Autodesk Inventor part; units mm, degrees
ref_plane "YZ Plane" through (0, 0, 0) normal (1, 0, 0) x (0, 1, 0)
ref_plane "XZ Plane" through (0, 0, 0) normal (0, 1, 0) x (-1, 0, 0)
ref_plane "XY Plane" through (0, 0, 0) normal (0, 0, 1) x (1, 0, 0)
sketch "스케치1" plane through (0, 0, 0) normal (0, 0, 1) x (1, 0, 0)
  line L0 (27.7299, -18.5773) -> (-27.7299, -18.5773)
  line L1 (-27.7299, -18.5773) -> (-27.7299, 18.5773)
  line L2 (-27.7299, 18.5773) -> (27.7299, 18.5773)
  line L3 (27.7299, 18.5773) -> (27.7299, -18.5773)
  line L4 (27.7299, -18.5773) -> (-27.7299, 18.5773) construction
  line L5 (-27.7299, -18.5773) -> (27.7299, 18.5773) construction
  point P0 (0, 0)
extrude "돌출1" add sketch "스케치1" along normal blind 10
sketch "스케치2" plane through (0, 0, 10) normal (0, 0, 1) x (1, 0, 0)
  line L0 (27.7299, 18.5773) -> (-27.7299, 18.5773)
  line L1 (-19.7299, 18.5773) -> (19.7299, 18.5773)
  line L2 (19.7299, 18.5773) -> (19.7299, 3.5485)
  line L3 (19.7299, 3.5485) -> (-19.7299, 3.5485)
  line L4 (-19.7299, 3.5485) -> (-19.7299, 18.5773)
  line L5 (27.7299, -18.5773) -> (27.7299, 18.5773)
  line L6 (-27.7299, 18.5773) -> (-27.7299, -18.5773)
  point P0 (0, 0)
  dimension "d2" = 8
  dimension "d3" = 8
sketch "스케치3" plane through (-27.7299, 18.5773, 0) normal (0, 1, 0) x (1, 0, 0)
  line L0 (0, -10) -> (55.4598, -10)
  line L1 (46.066, -10) -> (10.9091, -10)
  line L2 (10.9091, -10) -> (10.9091, -19.7265)
  line L3 (10.9091, -19.7265) -> (46.066, -19.7265)
  line L4 (46.066, -19.7265) -> (46.066, -10)
  circle A0 centre (28.4876, -32.3685) radius 21.7725
  point P0 (27.7299, 0)
extrude "돌출2" add sketch "스케치3" against normal blind 15
sketch "스케치4" plane through (-27.7299, 3.5773, 0) normal (0, -1, 0) x (1, 0, 0)
  circle A0 centre (28.6894, 33.7874) radius 10.835
  arc A1 (46.066, 19.5217) -> (10.9091, 19.5217) centre (28.4876, 32.3685) ccw
  arc A2 (46.2263, 44.9931) -> (36.5571, 52.5904) centre (41.9392, 49.4885) ccw
  arc A3 (21.0294, 52.8238) -> (10.3775, 44.4543) centre (15.036, 49.4885) ccw
  point P0 (27.7299, 0)
extrude "돌출3" add sketch "스케치4" along normal blind 20 contours A0
sketch "스케치5" plane through (-27.7299, 18.5773, 0) normal (0, 1, 0) x (1, 0, 0)
  arc A0 (10.9091, -19.5217) -> (46.066, -19.5217) centre (28.4876, -32.3685) ccw
  arc A1 (10.2823, -44.3105) -> (20.7748, -52.7291) centre (14.8621, -49.3505) ccw
  arc A2 (36.5162, -52.6067) -> (46.5049, -44.5922) centre (42.1131, -49.3505) ccw
  point P0 (27.7299, 0)
extrude "돌출4" add sketch "스케치5" against normal blind 10
properties part number "240626_part2"
The listing builds one solid part. Answer for the finished solid, in the listing's coordinates (mm). A direction names the side the tool comes from. Round coordinates to 2 decimals unless told otherwise and drop trailing zeros. Write each loop counter-clockwise with the first axis right and the second up, starting at its lowest first coordinate (ties: lowest second). Pieces come first, ordered by that corner, then holes. Notation, with made-up numbers: (55.25, 67) - (91.25, 67) arc R32 ccw to (91.25, 98) - close; hole circle Ø9 at (58, 75). An arc over 180 degrees is marked (long way). Use one line per item in the form item = value. Start each with the question number.
Item 1: Find the intervals of material crossed by line 1 (Z direction, x = -19, y = 3); line 2 (Y direction, x = 1, z = 17); line 3 (X direction, y = 16.5, z = 17.5), in increasing order. Write a range as [from, to].
Item 2: A tool of negligible diameter and unlimited length cuts with its end or side. For faces 1 (the cylindrical face through (-10.063, 7.849, 51.262)), 2 (the flat face through (-16.821, 11, 15)), 3 (the flat face through (1, -16.423, 34)), 4 (the flat face through (18.336, 11, 15)), from which of +Z, -Z, +X, -X, +Y, -Y can it reach the whole face along a straight path? Write none if from no direction.
Item 3: A cutting plane is placed at A-A (y = 5). Write down the section's boundary in (x, z) (1 decimal).
Item 4: A cutting plane is placed at B-B (z = 39). Write down the section's boundary in (x, y).
Item 5: Determine the mould class of faces 5 (the cylindrical face through (-17.257, 13.647, 54.557)), 6 (the flat face through (27.73, 0, 5)), 7 (the flat face through (0, 0, 0)) for opening direction Z: +Z half, -Z half, draft (parallel to the pull), parting line (faces both ways), or undercut.
Item 6: A cutting plane is placed at C-C (x = 0). Write down the section's boundary in (y, z), plus the area to 3 significant figures.
Item 7: Flat-ended cylindrical pins translate along their axes: pin 1 Ø7.5 at (y, z) = (9, 16) entering from -X; pin 2 Ø6.5 at (x, z) = (0.5, 30.5) entering from -Y; pin 3 Ø6 at (y, z) = (7, 32.5) entering from +X. Find the tip coordinate at first contact, or state that the pin passes through.
Item 8: A cutting plane is placed at D-D (y = -6.5). Write down the section's boundary in (x, z) (1 decimal).
The answers:
q1.line_1 = [0, 10]
q1.line_2 = [3.58, 18.58]
q1.line_3 = [-16.82, 18.34]
q2.face_1 = -Y
q2.face_2 = -X, +Y, -Y
q2.face_3 = +Z, +X, -X, -Y
q2.face_4 = +X, +Y, -Y
q3.outline = (-27.7, 0) - (27.7, 0) - (27.7, 10) - (18.3, 10) - (18.3, 19.5) arc R21.8 ccw (long way) to (-16.8, 19.5) - (-16.8, 10) - (-27.7, 10) - close
q4.outline = (-19.98, 3.58) - (-8.54, 3.58) - (-8.54, -16.42) - (10.46, -16.42) - (10.46, 3.58) - (21.5, 3.58) - (21.5, 18.58) - (-19.98, 18.58) - close
q5.face_5 = undercut
q5.face_6 = draft
q5.face_7 = -Z half
q6.outline = (-18.58, 0) - (18.58, 0) - (18.58, 54.13) - (3.58, 54.13) - (3.58, 44.58) - (-16.42, 44.58) - (-16.42, 22.99) - (3.58, 22.99) - (3.58, 10) - (-18.58, 10) - close
q6.area = 1,470 mm^2
q7.pin_1 = -16.99
q7.pin_2 = -16.42
q7.pin_3 = 22.53
q8.outline = (-27.7, 0) - (27.7, 0) - (27.7, 10) - (-27.7, 10) - close; circle Ø21.7 at (1, 33.8)
